Geometry check sheet. Reference: drawing and pictorial views, mm from the part's lowest x, y, z. A direction names the side the tool comes from. Give positions to 0.01 mm unless a question says otherwise; leave off trailing zeros. Order: outer loops, then holes, each group sorted by start corner. A loop starts at its lowest first (then second) coordinate and runs counter-clockwise, first axis right, second up.
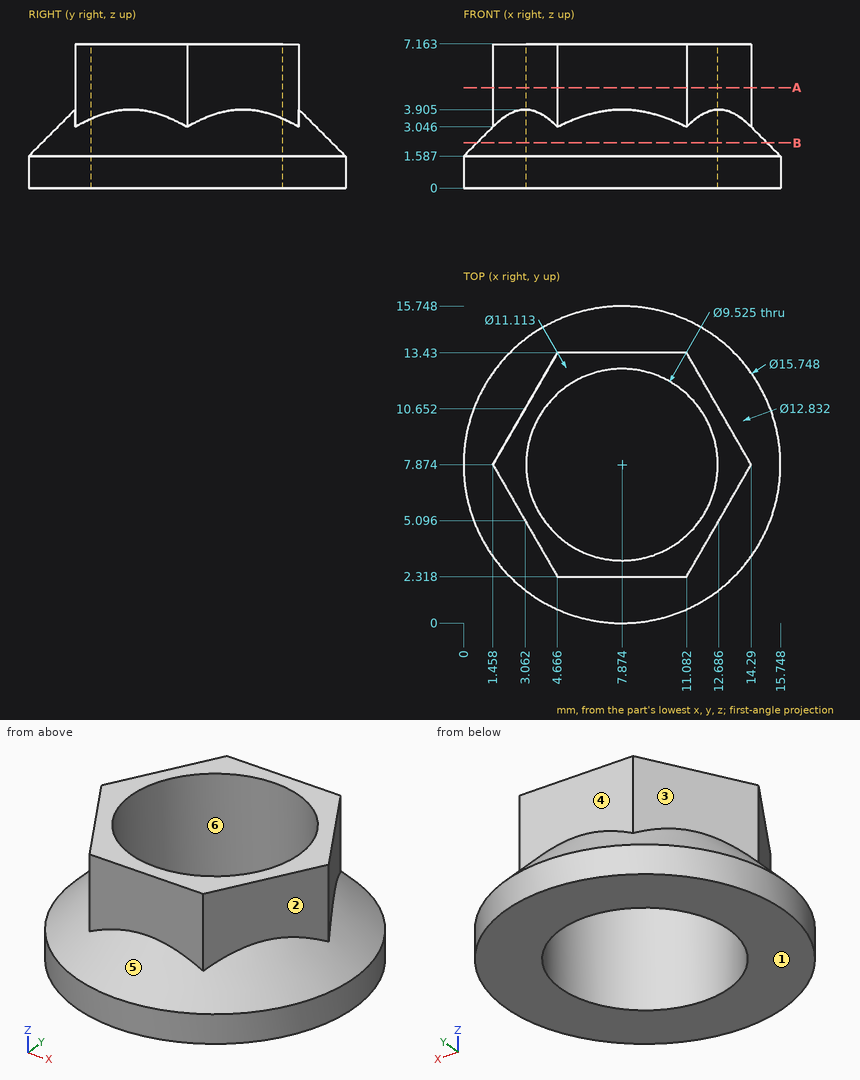
1) Section check B-B, the plane z = 2.25. Record the cut outline in (x, y) (1 decimal).
Recorded:
outline: circle Ø14.4 at (7.9, 7.9); hole circle Ø9.5 at (7.9, 7.9)
2) Set-up check for the marked faces 1, 2 and 3: record each of +Z, -Z, +X, -X, +Y, -Y from which the full face is reachable in a straight line by a thin tool's end or side.
Recorded:
face 1: -Z, +X, -X, +Y, -Y
face 2: +Z, +X, -Y
face 3: +Z, -X, +Y
3) Section check A-A, the plane z = 5. Record the cut outline in (x, y) (1 decimal).
Recorded:
outline: (1.5, 7.9) - (4.7, 2.3) - (11.1, 2.3) - (14.3, 7.9) - (11.1, 13.4) - (4.7, 13.4) - close; hole circle Ø9.5 at (7.9, 7.9)
4) Material ranges on L1, parallel to X at y = 9.25, z = 3.25 (1 decimal); L2, parallel to Y at x = 6, z = 4.75 (1 decimal); L3, parallel to X at y = 5, z = 3 (1 decimal), recorded low to high.
Recorded:
L1: x = 1.8 to 3.3, 12.4 to 13.9
L2: y = 2.3 to 3.5, 12.3 to 13.4
L3: x = 2.1 to 4.1, 11.7 to 13.7
5) Draft check along Y on the marked faces 4, 5 and 6. Enter one of: +Y half, -Y half, draft (parallel to the pull), parting line (faces both ways), or undercut.
Recorded:
face 4: +Y half
face 5: parting line
face 6: undercut
6) Depth check by flat-ended pin: pin 1 Ø2 at (x, z) = (12, 3) entering from -Y (1 decimal); pin 2 Ø4 at (x, z) = (11.5, 4.5) entering from -Y (1 decimal); pin 3 Ø2 at (x, z) = (7, 5.5) entering from -Y. Enter the tip coordinate at first touch or a pass-through.
Recorded:
pin 1: stops at y = 1.5
pin 2: stops at y = 1.7
pin 3: stops at y = 2.32
